Autodesk Inventor part; units mm, degrees
ref_plane "YZ Plane" through (0, 0, 0) normal (1, 0, 0) x (0, 1, 0)
ref_plane "XZ Plane" through (0, 0, 0) normal (0, 1, 0) x (-1, 0, 0)
ref_plane "XY Plane" through (0, 0, 0) normal (0, 0, 1) x (1, 0, 0)
sketch "Sketch1" plane through (0, 0, 0) normal (0, 1, 0) x (-1, 0, 0)
  line L0 (106.9403, 291.2572) -> (195.8403, 291.2572)
  line L1 (202.1903, 284.9072) -> (202.1903, 94.4072)
  line L2 (195.8403, 88.0572) -> (106.9403, 88.0572)
  line L3 (100.5903, 94.4072) -> (100.5903, 284.9072)
  arc A0 (202.1903, 284.9072) -> (195.8403, 291.2572) centre (195.8403, 284.9072) ccw
  arc A1 (195.8403, 88.0572) -> (202.1903, 94.4072) centre (195.8403, 94.4072) ccw
  arc A2 (106.9403, 291.2572) -> (100.5903, 284.9072) centre (106.9403, 284.9072) ccw
  arc A3 (100.5903, 94.4072) -> (106.9403, 88.0572) centre (106.9403, 94.4072) ccw
  line L4 (200.3304, 289.3973) -> (236.2514, 325.3183)
  line L5 (200.3304, 289.3973) -> (251.1304, 289.3973) construction
  line L6 (200.3304, 89.917) -> (236.2514, 53.996)
  line L7 (200.3304, 89.917) -> (251.1304, 89.917) construction
  line L8 (102.4502, 289.3973) -> (66.5291, 325.3183) construction
  line L9 (102.4502, 89.917) -> (66.5291, 53.996)
  line L10 (102.4502, 89.917) -> (153.2502, 89.917) construction
  arc A4 (228.2944, 301.1968) -> (212.13, 317.3613) centre (236.2514, 325.3183) ccw
  circle A5 centre (236.2514, 53.996) radius 25.4
  arc A6 (90.6506, 317.3613) -> (74.4862, 301.1968) centre (66.5291, 325.3183) ccw
  circle A7 centre (66.5291, 53.996) radius 25.4
  line L11 (66.5291, 325.3183) -> (58.4469, 317.2361)
  line L12 (58.4469, 317.2361) -> (100.5903, 275.0927)
  line L13 (66.5291, 325.3183) -> (74.6114, 333.4006)
  line L14 (74.6114, 333.4006) -> (116.7547, 291.2572)
  line L15 (236.2514, 325.3183) -> (228.1692, 333.4006)
  line L16 (228.1692, 333.4006) -> (236.2514, 325.3183)
  line L17 (236.2514, 325.3183) -> (244.3337, 317.2361)
  line L18 (228.1692, 333.4006) -> (186.0258, 291.2572)
  line L19 (244.3337, 317.2361) -> (202.1903, 275.0927)
  line L20 (293.8482, 183.4348) -> (-26.9886, 183.4348) construction
  line L21 (236.2514, 53.996) -> (228.1692, 45.9138)
  line L22 (236.2514, 53.996) -> (247.6814, 53.996) construction
  line L23 (236.2514, 53.996) -> (244.3337, 62.0783)
  line L24 (228.1692, 45.9138) -> (186.0258, 88.0572)
  line L25 (244.3337, 62.0783) -> (202.1903, 104.2216)
  line L26 (66.5291, 53.996) -> (74.6114, 45.9138)
  line L27 (66.5291, 53.996) -> (58.4469, 62.0783)
  line L28 (58.4469, 62.0783) -> (100.5903, 104.2216)
  line L29 (74.6114, 45.9138) -> (116.7547, 88.0572)
  circle A8 centre (66.5291, 325.3183) radius 25.4
  circle A9 centre (236.2514, 325.3183) radius 25.4
  line L30 (66.5291, 325.3183) -> (102.4502, 289.3973)
  point P0 (0, 0)
  point P1 (202.1903, 88.0572)
  point P2 (202.1903, 291.2572)
  point P3 (100.5903, 88.0572)
  point P4 (228.2944, 78.1175)
  point P5 (212.13, 61.953)
  point P6 (74.4862, 78.1175)
  point P7 (90.6506, 61.953)
  point P8 (74.4862, 301.1968)
  dimension "d0" = 101.6
  dimension "d1" = 203.2
  dimension "d2" = 6.35
  dimension "d3" = 50.8
  dimension "d4" = 45
  dimension "d5" = 50.8
  dimension "d6" = 45
  dimension "d7" = 50.8
  dimension "d8" = 50.8
  dimension "d9" = 135
  dimension "d10" = 50.8
  dimension "d11" = 50.8
  dimension "d12" = 50.8
  dimension "d13" = 50.8
  dimension "d14" = 11.43
  dimension "d15" = 11.43
  dimension "d16" = 11.43
  dimension "d17" = 135
  dimension "d18" = 11.43
  dimension "d19" = 11.43
  dimension "d20" = 11.43
extrude "Extrusion1" add sketch "Sketch1" along normal blind 101.6 contours L0 A0 L1 A1 L2 A3 L3 A2
extrude "Extrusion2" add sketch "Sketch1" along normal blind 101.6 contours A2 L30 A8 L14 L0 | A2 L3 L12 A8 L30 | L18 A9 L4 A0 L0 | L14 L13 L11 L12 A6 | A8 L30 L13 L14 | A8 L12 L11 L30 | A4 L19 L17 L15 L18 | L18 L15 L4 A9 | L4 A9 L19 L1 A0 | L4 L17 L19 A9 | L3 A3 L9 A7 L28 | L28 L27 L26 L29 A7 | A7 L9 L27 L28 | A3 L2 L29 A7 L9 | A7 L29 L26 L9 | L25 A5 L6 A1 L1 | L25 L23 L6 A5 | A5 L24 L21 L23 L25 | L6 A5 L24 L2 A1 | L6 L21 L24 A5
extrude "Extrusion3" cut sketch "Sketch1" along normal blind 38.1 contours A2 L30 A8 L14 L0 | A2 L3 L12 A8 L30
sketch "Sketch2" plane through (0, 101.6, 0) normal (0, 1, 0) x (1, 0, 0)
  line L0 (106.9403, 291.2572) -> (195.8403, 291.2572)
  line L1 (202.1903, 284.9072) -> (202.1903, 94.4072)
  line L2 (195.8403, 88.0572) -> (106.9403, 88.0572)
  line L3 (100.5903, 94.4072) -> (100.5903, 284.9072)
  arc A0 (202.1903, 284.9072) -> (195.8403, 291.2572) centre (195.8403, 284.9072) ccw
  arc A1 (195.8403, 88.0572) -> (202.1903, 94.4072) centre (195.8403, 94.4072) ccw
  arc A2 (106.9403, 291.2572) -> (100.5903, 284.9072) centre (106.9403, 284.9072) ccw
  arc A3 (100.5903, 94.4072) -> (106.9403, 88.0572) centre (106.9403, 94.4072) ccw
  line L4 (200.3304, 289.3973) -> (236.2514, 325.3183)
  line L5 (200.3304, 289.3973) -> (251.1304, 289.3973) construction
  line L6 (200.3304, 89.917) -> (236.2514, 53.996)
  line L7 (200.3304, 89.917) -> (251.1304, 89.917) construction
  line L8 (102.4502, 289.3973) -> (66.5291, 325.3183) construction
  line L9 (102.4502, 89.917) -> (66.5291, 53.996)
  line L10 (102.4502, 89.917) -> (153.2502, 89.917) construction
  arc A4 (228.2944, 301.1968) -> (212.13, 317.3613) centre (236.2514, 325.3183) ccw
  circle A5 centre (236.2514, 53.996) radius 25.4
  arc A6 (90.6506, 317.3613) -> (74.4862, 301.1968) centre (66.5291, 325.3183) ccw
  circle A7 centre (66.5291, 53.996) radius 25.4
  line L11 (66.5291, 325.3183) -> (58.4469, 317.2361)
  line L12 (58.4469, 317.2361) -> (100.5903, 275.0927)
  line L13 (66.5291, 325.3183) -> (74.6114, 333.4006)
  line L14 (74.6114, 333.4006) -> (116.7547, 291.2572)
  line L15 (236.2514, 325.3183) -> (228.1692, 333.4006)
  line L16 (228.1692, 333.4006) -> (236.2514, 325.3183)
  line L17 (236.2514, 325.3183) -> (244.3337, 317.2361)
  line L18 (228.1692, 333.4006) -> (186.0258, 291.2572)
  line L19 (244.3337, 317.2361) -> (202.1903, 275.0927)
  line L20 (293.8482, 183.4348) -> (-26.9886, 183.4348) construction
  line L21 (236.2514, 53.996) -> (228.1692, 45.9138)
  line L22 (236.2514, 53.996) -> (247.6814, 53.996) construction
  line L23 (236.2514, 53.996) -> (244.3337, 62.0783)
  line L24 (228.1692, 45.9138) -> (186.0258, 88.0572)
  line L25 (244.3337, 62.0783) -> (202.1903, 104.2216)
  line L26 (66.5291, 53.996) -> (74.6114, 45.9138)
  line L27 (66.5291, 53.996) -> (58.4469, 62.0783)
  line L28 (58.4469, 62.0783) -> (100.5903, 104.2216)
  line L29 (74.6114, 45.9138) -> (116.7547, 88.0572)
  circle A8 centre (66.5291, 325.3183) radius 25.4
  circle A9 centre (236.2514, 325.3183) radius 25.4
  line L30 (66.5291, 325.3183) -> (102.4502, 289.3973)
  line L31 (200.3304, 289.3973) -> (102.4502, 89.917)
  line L32 (200.3304, 89.917) -> (102.4502, 289.3973)
  point P0 (0, 0)
  point P1 (202.1903, 88.0572)
  point P2 (202.1903, 291.2572)
  point P3 (100.5903, 88.0572)
  point P4 (228.2944, 78.1175)
  point P5 (212.13, 61.953)
  point P6 (74.4862, 78.1175)
  point P7 (90.6506, 61.953)
  point P8 (74.4862, 301.1968)
  dimension "d27" = 101.6
  dimension "d28" = 203.2
  dimension "d29" = 6.35
  dimension "d30" = 50.8
  dimension "d31" = 45
  dimension "d32" = 50.8
  dimension "d33" = 45
  dimension "d34" = 50.8
  dimension "d35" = 50.8
  dimension "d36" = 135
  dimension "d37" = 50.8
  dimension "d38" = 50.8
  dimension "d39" = 50.8
  dimension "d40" = 50.8
  dimension "d41" = 11.43
  dimension "d42" = 11.43
  dimension "d43" = 11.43
  dimension "d44" = 135
  dimension "d45" = 11.43
  dimension "d46" = 11.43
  dimension "d47" = 11.43
Design review of the part built by this model. Coordinates are the model's own, in mm. A direction names the side the tool comes from. Round coordinates to 2 decimals unless told otherwise and drop trailing zeros. Write each loop counter-clockwise with the first axis right and the second up, starting at its lowest first coordinate (ties: lowest second). Pieces come first, ordered by that corner, then holes. Notation, with made-up numbers: (27.25, -11.5) - (36.25, -11.5) arc R11 ccw to (36.25, -7.5) - close; hole circle Ø10 at (-10, 54). An arc over 180 degrees is marked (long way). Use a Markdown table: item, result. Add a question column.
1. We need section A-A (z = 305.5). State the section outline as (x, y) points.
2. We need section C-C (x = -122.5). State the section outline as (y, z) points.
3. We need section B-B (y = 20). State the section outline as (x, z) points.
4. We need section D-D (z = 137.5). State the section outline as (x, y) points.
5. For faces 4 (the face through (-253.527, 50.089, 343.939)), 5 (the face through (-152, 50, 88.057)), 6 (the face through (-95, 38.1, 297)), list the 3-axis set-ups (+Z, -Z, +X, -X, +Y, -Y) from which the entire face can be reached by the end or side of a thin tool; tool diameter is ignored.
6. Mouldability with a two-part tool opening along X and no side actions: class faces 1 (the face through (-102.401, 18.783, 289.348)), 2 (the face through (-47.909, 50.089, 342.594)), 3 (the face through (-150, 101.6, 192)) as +X half, -X half, draft (parallel to the pull), parting line (faces both ways), or undercut.
7. Wall thickness on probe 1 along X at (y, z) = (57, 130); probe 2 along X at (y, z) = (71, 75); probe 3 along Z at (x, y) = (-246.5, 12): over which ranges is each line inside the solid? List them lowest first.
8. Clearance check with flat-ended pins moving along their axes: pin 1 (10 mm diameter, centred on y = 65.5, z = 242.5, fed in from +X); pin 2 (10 mm diameter, centred on y = 45.5, z = 166, fed in from -X); pin 3 (4 mm diameter, centred on y = 64.5, z = 96, fed in from +X). State where each tip first meets the part, or that it passes through.
Output:
| question | item | result |
|---|---|---|
| 1 | outline | (-252.14, 0) - (-200.27, 0) - (-200.27, 101.6) - (-252.14, 101.6) - close; (-102.51, 38.1) - (-82.42, 38.1) - (-82.42, 0) - (-50.64, 0) - (-50.64, 101.6) - (-102.51, 101.6) - close |
| 2 | outline | (0, 88.06) - (101.6, 88.06) - (101.6, 291.26) - (0, 291.26) - close |
| 3 | outline | (-228.29, 78.12) arc R25.4 ccw (long way) to (-212.13, 61.95) - (-186.03, 88.06) - (-116.75, 88.06) - (-90.65, 61.95) arc R25.4 ccw (long way) to (-74.49, 78.12) - (-100.59, 104.22) - (-100.59, 284.91) arc R6.35 ccw to (-106.94, 291.26) - (-186.03, 291.26) - (-212.13, 317.36) arc R25.4 ccw (long way) to (-228.29, 301.2) - (-202.19, 275.09) - (-202.19, 104.22) - close; (-90.65, 317.36) arc R25.4 ccw to (-74.49, 301.2) arc R25.4 ccw (long way) to start |
| 4 | outline | (-202.19, 0) - (-100.59, 0) - (-100.59, 101.6) - (-202.19, 101.6) - close |
| 5 | face 4 | +Y, -Y |
| 5 | face 5 | -Z, +Y, -Y |
| 5 | face 6 | -Y |
| 6 | face 1 | +X half |
| 6 | face 2 | undercut |
| 6 | face 3 | draft |
| 7 | probe 1 | x = -202.19 to -100.59 |
| 7 | probe 2 | x = -250.53 to -199.08, -103.7 to -52.25 |
| 7 | probe 3 | z = 30.76 to 77.24, 302.08 to 348.56 |
| 8 | pin 1 | stops at x = -100.59 |
| 8 | pin 2 | stops at x = -202.19 |
| 8 | pin 3 | stops at x = -90.37 |
